The drawing under review shows one solid part. Ordinate dimensions are in mm from its lowest x, y, z. A direction names the side the tool comes from. Coordinates: 2 decimals unless noted, no trailing zeros. Loops run counter-clockwise (first coordinate to the right, second up) from the corner with the lowest first, then second, coordinate; pieces in that order, holes last.
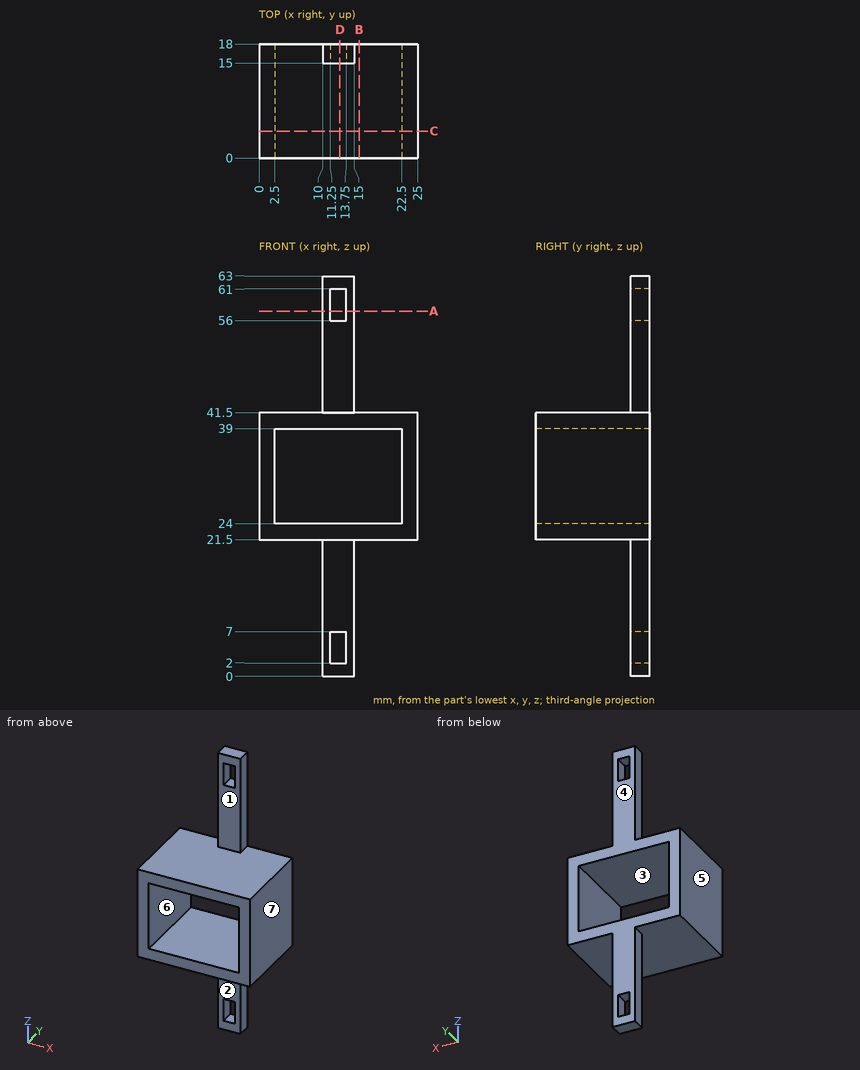
Q1. Machinability: for the marked faces 1, 2, 3 and 4, which of the approach directions +Z, -Z, +X, -X, +Y, -Y give a long, thin tool a straight path to every point of the face, cutting with its end or side? Answer none if there is none.
Q2. For line 1 (Z direction, x = 8.5, y = 10); line 2 (X direction, y = 6, z = 33); line 3 (X direction, y = 16, z = 57), list the stretches that pass through material, from the lowest coordinate up.
Q3. Take a section at B-B, the plane x = 15.75. Write out the cut boundary in (y, z).
Q4. The part is to be moulded in two halves that separate along X. For the marked faces 5, 6 and 7, say which applies: pulls with the +X half, pulls with the -X half, needs draft (parallel to the pull), parting line crosses it, or undercut.
Q5. Take a section at C-C, the plane y = 4.25. Write out the cut boundary in (x, z).
Q6. Take a section at D-D, the plane x = 12.75. Write out the cut boundary in (y, z).
Q7. Clearance check with flat-ended pins moving along their axes: pin 1 Ø9 at (x, y) = (16.5, 5) entering from +Z; pin 2 Ø1.5 at (x, z) = (12.5, 13) entering from -Y; pin 3 Ø2.5 at (y, z) = (16.5, 50) entering from -X. State where each tip first meets the part, or that it passes through.
Q8. Take a section at A-A, the plane z = 57.5. Write out the cut boundary in (x, y).
Entries:
1. face 1: +Z, +X, -X, -Y
1. face 2: -Z, +X, -X, -Y
1. face 3: +Y, -Y
1. face 4: +Z, -Z, +X, -X, +Y
2. line 1: z = 21.5 to 24, 39 to 41.5
2. line 2: x = 0 to 2.5, 22.5 to 25
2. line 3: x = 10 to 11.25, 13.75 to 15
3. outline: (0, 21.5) - (18, 21.5) - (18, 24) - (0, 24) - close; (0, 39) - (18, 39) - (18, 41.5) - (0, 41.5) - close
4. face 5: pulls with the -X half
4. face 6: undercut
4. face 7: pulls with the +X half
5. outline: (0, 21.5) - (25, 21.5) - (25, 41.5) - (0, 41.5) - close; hole (2.5, 24) - (22.5, 24) - (22.5, 39) - (2.5, 39) - close
6. outline: (0, 21.5) - (15, 21.5) - (15, 7) - (18, 7) - (18, 24) - (0, 24) - close; (0, 39) - (18, 39) - (18, 56) - (15, 56) - (15, 41.5) - (0, 41.5) - close; (15, 0) - (18, 0) - (18, 2) - (15, 2) - close; (15, 61) - (18, 61) - (18, 63) - (15, 63) - close
7. pin 1: stops at z = 41.5
7. pin 2: stops at y = 15
7. pin 3: stops at x = 10
8. outline: (10, 15) - (11.25, 15) - (11.25, 18) - (10, 18) - close; (13.75, 15) - (15, 15) - (15, 18) - (13.75, 18) - close
